Part print with two shaded views. Sizes in mm from the minimum x, y, z corner. A direction names the side the tool comes from. Coordinates: 2 decimals unless noted, no trailing zeros. Order: outer loops, then holes, each group sorted by start corner. A loop starts at its lowest first (then second) coordinate and runs counter-clockwise, first axis right, second up. Notation, with made-up numbers: M 41.5,-15 L 74.5,-15 A24 ccw 74.5,24 Z; hole C 35,48.25 d3. An arc over 180 degrees is marked long. Answer in a Markdown table with one row per item. Add a question column.
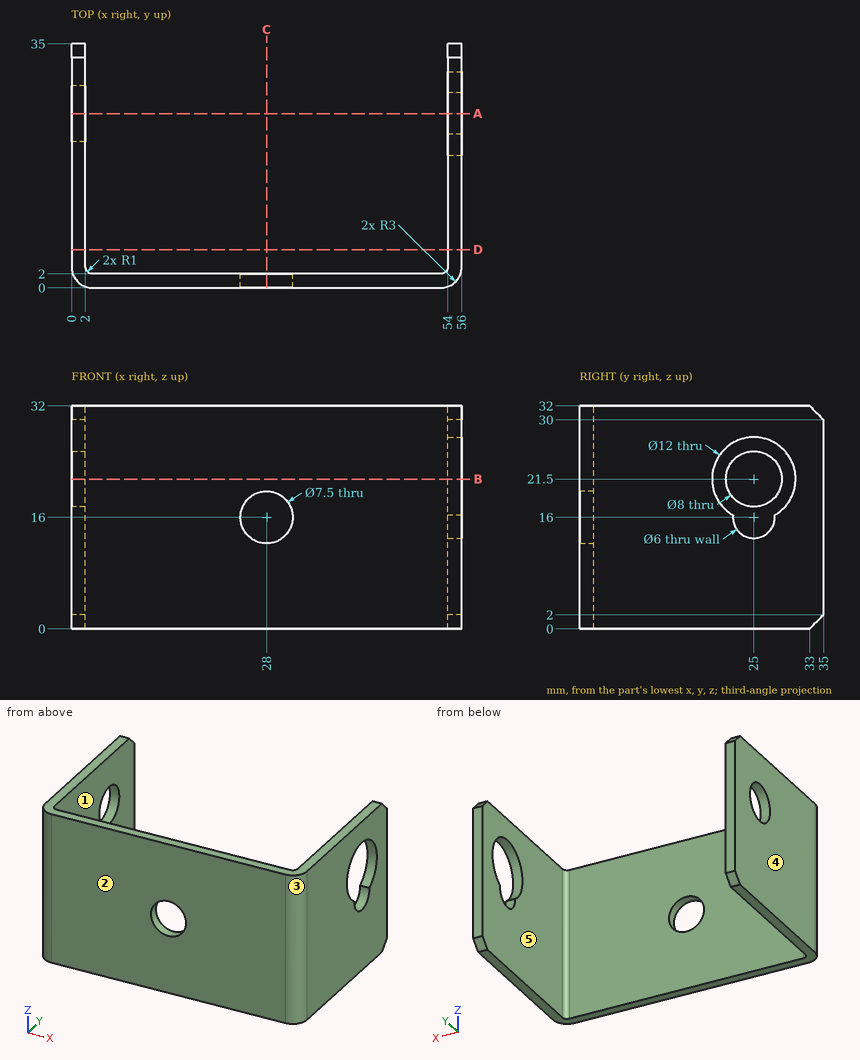
(1) Slice it at B-B (z = 21.5). List the corners of the cut face in (x, y), and give its area (3 significant figures).
(2) Drop flat-ended pins along their axis: P1, Ø5, axis at y = 25, z = 21.5, coming from the -X side; P2, Ø3, axis at x = 13.5, z = 13, coming from the +Y side. Give the stop position or say it passes through.
(3) Slice it at C-C (x = 28). List the corners of the cut face in (y, z), and give its area (3 significant figures).
(4) Slice it at A-A (y = 25). List the corners of the cut face in (x, z), and give its area (3 significant figures).
(5) Wall check: line 1 (X direction, y = 5, z = 3); line 2 (Y direction, x = 18, z = 11); line 3 (X direction, y = 1.5, z = 16). Give the ranges that are in metal, low to high.
(6) Pull direction X, two halves, no side cores. Call the marked faces 3, 4 and 5: pulls with the +X half, pulls with the -X half, needs draft (parallel to the pull), parting line crosses it, or undercut.
(7) Slice it at D-D (y = 5.5). List the corners of the cut face in (x, z), and give its area (3 significant figures).
(8) 3-axis set-ups, long thin cutter, end or side, ignore diameter. For the marked faces 1 and 2: which of +Z, -Z, +X, -X, +Y, -Y reach the whole face in a straight line?
Computed:
| question | item | result |
|---|---|---|
| 1 | outline | M 0,3 A3 ccw 3,0 L 53,0 A3 ccw 56,3 L 56,19 L 54,19 L 54,3 A1 cw 53,2 L 3,2 A1 cw 2,3 L 2,21 L 0,21 Z; M 0,29 L 2,29 L 2,35 L 0,35 Z; M 54,31 L 56,31 L 56,35 L 54,35 Z |
| 1 | area | 201 mm^2 |
| 2 | P1 | passes through |
| 2 | P2 | stops at y = 2 |
| 3 | outline | M 0,0 L 2,0 L 2,12.25 L 0,12.25 Z; M 0,19.75 L 2,19.75 L 2,32 L 0,32 Z |
| 3 | area | 49.0 mm^2 |
| 4 | outline | M 0,0 L 2,0 L 2,17.5 L 0,17.5 Z; M 0,25.5 L 2,25.5 L 2,32 L 0,32 Z; M 54,0 L 56,0 L 56,13 L 54,13 Z; M 54,27.5 L 56,27.5 L 56,32 L 54,32 Z |
| 4 | area | 83.0 mm^2 |
| 5 | line 1 | x = 0 to 2, 54 to 56 |
| 5 | line 2 | y = 0 to 2 |
| 5 | line 3 | x = 0.4 to 24.25, 31.75 to 55.6 |
| 6 | face 3 | pulls with the +X half |
| 6 | face 4 | pulls with the -X half |
| 6 | face 5 | undercut |
| 7 | outline | M 0,0 L 2,0 L 2,32 L 0,32 Z; M 54,0 L 56,0 L 56,32 L 54,32 Z |
| 7 | area | 128 mm^2 |
| 8 | face 1 | +Z, -Z, +Y |
| 8 | face 2 | +Z, -Z, +X, -X, -Y |
